Autodesk Inventor part; units mm, degrees
ref_plane "YZ Plane" through (0, 0, 0) normal (1, 0, 0) x (0, 1, 0)
ref_plane "XZ Plane" through (0, 0, 0) normal (0, 1, 0) x (-1, 0, 0)
ref_plane "XY Plane" through (0, 0, 0) normal (0, 0, 1) x (1, 0, 0)
sketch "Sketch1" plane through (0, 0, 0) normal (0, 0, 1) x (1, 0, 0)
  circle A0 centre (0, 0) radius 31
  circle A1 centre (0, 0) radius 34.175
  dimension "d0" = 62
  dimension "d1" = 68.35
extrude "Extrusion1" add sketch "Sketch1" along normal blind 6.35
ref_plane "Work Plane1" through (0, 0, -83.5) normal (0, 0, -1) x (-1, 0, 0)
sketch "Sketch2" plane through (0, 0, -83.5) normal (0, 0, -1) x (-1, 0, 0)
  circle A0 centre (0, 0) radius 30
  circle A1 centre (0, 0) radius 33.175
  circle A2 centre (0, 0) radius 23
  circle A3 centre (0, 0) radius 26.175
  dimension "d5" = 60
  dimension "d6" = 66.35
  dimension "d28" = 46
  dimension "d29" = 52.35
ref_plane "Work Plane2" through (0, 0, -57.65) normal (0, 0, -1) x (-1, 0, 0)
sketch "Sketch3" plane through (0, 0, -57.65) normal (0, 0, -1) x (-1, 0, 0)
  circle A0 centre (0, 0) radius 34.175
  circle A1 centre (0, 0) radius 31
  circle A2 centre (0, 0) radius 24
  circle A3 centre (0, 0) radius 27.175
  line L0 (0, 0) -> (34.175, 0)
  line L1 (0, 0) -> (34.175, 0) construction
  line L2 (0, 0) -> (33.8826, 4.4607)
  line L3 (0, 0) -> (33.8826, -4.4607)
  line L4 (33.8826, 4.4607) -> (33.8826, -4.4607)
  line L5 (33.8826, -4.4607) -> (0, -4.4607)
  line L6 (0, -4.4607) -> (0, 4.4607)
  line L7 (0, 4.4607) -> (33.8826, 4.4607)
  line L8 (33.8826, 4.4607) -> (33.8826, -4.4607)
  line L9 (33.8826, -4.4607) -> (37.0576, -4.4607)
  line L10 (37.0576, -4.4607) -> (37.0576, 4.4607)
  line L11 (37.0576, 4.4607) -> (33.8826, 4.4607)
  line L12 (-3.8631, 2.2304) -> (13.0782, 31.5736)
  line L13 (20.8044, 27.1129) -> (3.8631, -2.2304)
  line L14 (20.8044, 27.1129) -> (22.3919, 29.8625)
  line L15 (14.6657, 34.3232) -> (13.0782, 31.5736)
  line L16 (-3.8631, -2.2304) -> (-20.8044, 27.1129)
  line L17 (-13.0782, 31.5736) -> (3.8631, 2.2304)
  line L18 (-13.0782, 31.5736) -> (-14.6657, 34.3232)
  line L19 (-22.3919, 29.8625) -> (-20.8044, 27.1129)
  line L20 (0, -4.4607) -> (-33.8826, -4.4607)
  line L21 (-33.8826, 4.4607) -> (0, 4.4607)
  line L22 (-33.8826, 4.4607) -> (-37.0576, 4.4607)
  line L23 (-37.0576, -4.4607) -> (-33.8826, -4.4607)
  line L24 (3.8631, -2.2304) -> (-13.0782, -31.5736)
  line L25 (-20.8044, -27.1129) -> (-3.8631, 2.2304)
  line L26 (-20.8044, -27.1129) -> (-22.3919, -29.8625)
  line L27 (-14.6657, -34.3232) -> (-13.0782, -31.5736)
  line L28 (3.8631, 2.2304) -> (20.8044, -27.1129)
  line L29 (13.0782, -31.5736) -> (-3.8631, -2.2304)
  line L30 (13.0782, -31.5736) -> (14.6657, -34.3232)
  line L31 (22.3919, -29.8625) -> (20.8044, -27.1129)
  line L32 (-34.175, 6.35) -> (0, 6.35)
  line L33 (0, 6.35) -> (0, -6.35)
  line L34 (0, -6.35) -> (-34.175, -6.35)
  line L35 (-34.175, -6.35) -> (-34.175, 6.35)
  line L36 (-9.525, 34.175) -> (9.525, 34.175)
  line L37 (9.525, 34.175) -> (9.525, 0)
  line L38 (9.525, 0) -> (-9.525, 0)
  line L39 (-9.525, 0) -> (-9.525, 34.175)
  point P0 (-26.8064, 4.4607)
  point P1 (-33.8826, 4.4607)
  point P2 (-33.8826, -4.4607)
  point P3 (-26.8064, -4.4607)
  point P4 (-17.2663, -20.9846)
  point P5 (-20.8044, -27.1129)
  point P6 (-13.0782, -31.5736)
  point P7 (-9.5401, -25.4454)
  point P8 (9.5401, -25.4454)
  point P9 (20.8044, -27.1129)
  point P10 (17.2663, -20.9846)
  point P11 (26.8064, -4.4607)
  point P12 (26.8064, 4.4607)
  point P13 (17.2663, 20.9846)
  point P14 (20.8044, 27.1129)
  point P15 (13.0782, 31.5736)
  point P16 (9.5401, 25.4454)
  point P17 (-13.0782, 31.5736)
  point P18 (-20.8044, 27.1129)
  point P19 (-17.2663, 20.9846)
  point P20 (-9.5401, 25.4454)
  point P21 (-34.175, 0)
  point P22 (0, 0)
  point P23 (0, 0)
  point P24 (-7.9278, 22.6528)
  point P25 (-9.525, 25.4192)
  point P26 (-9.525, 29.5004)
  point P27 (9.525, 29.5004)
  point P28 (9.525, 25.4192)
  point P29 (7.9278, 22.6528)
  point P30 (-9.525, 22.0289)
  point P31 (9.525, 22.0289)
  dimension "d8" = 68.35
  dimension "d9" = 62
  dimension "d10" = 48
  dimension "d11" = 54.35
  dimension "d12" = 0
  dimension "d13" = 7.5
  dimension "d14" = 7.5
  dimension "d15" = 3.175
  dimension "d18" = 360
  dimension "d70" = 12.7
  dimension "d71" = 19.05
  dimension "d72" = 9.525
extrude "Extrusion2" add sketch "Sketch3" against normal up to surface (57.65 mm away) contours L0 L4 A0 | A0 L4 L0 | L7 A1 L13 A0 | L4 L0 A1 L2 | L2 A1 L7 | L5 A1 L3 | L3 A1 L0 L4 | A0 L28 A1 L5 | L13 A1 L12 A0 | A0 L29 A1 L28 | L12 A1 L37 A0 | A0 L24 A1 L29 | L37 A1 L39 A0 | A0 L25 A1 L24 | A0 L34 A1 L25 | L39 A1 L17 A0 | A0 L20 A1 L34 | L17 A1 L16 A0 | A0 L21 A1 L20 | L16 A1 L32 A0 | L32 A1 L21 A0
extrude "Extrusion3" add sketch "Sketch3" along normal blind 17 contours L2 A3 L7 A1 | A1 L0 A3 L2 | L7 A3 L13 A1 | L3 A3 L0 A1 | A1 L5 A3 L3 | A1 L28 A3 L5 | L13 A3 L12 A1 | L2 A2 L7 A3 | A3 L0 A2 L2 | L7 A2 L13 A3 | A1 L29 A3 L28 | L3 A2 L0 A3 | A3 L5 A2 L3 | A3 L28 A2 L5 | L12 A3 L37 A1 | L13 A2 L37 L12 A3 | A1 L24 A3 L29 | A3 L29 A2 L28 | L12 L37 A3 | A1 L25 A3 L24 | A3 L24 A2 L29 | L39 A3 L17 A1 | A1 L34 A3 L25 | A3 L25 A2 L24 | L17 A3 L16 A1 | L39 L17 A3 | A1 L20 A3 L34 | A3 L34 A2 L25 | L16 A3 L32 A1 | L17 L39 A2 L16 A3 | A1 L21 A3 L20 | A3 L20 A2 L34 | L32 A3 L21 A1 | L16 A2 L32 A3 | A3 L21 A2 L20 | L32 A2 L21 A3
extrude "Extrusion5" add sketch "Sketch3" along normal blind 6.35 contours L0 L4 A0 | A0 L4 L0 | L7 A1 L13 A0 | L4 L0 A1 L2 | L2 A1 L7 | L5 A1 L3 | L3 A1 L0 L4 | A0 L28 A1 L5 | L13 A1 L12 A0 | A0 L29 A1 L28 | L12 A1 L37 A0 | A0 L24 A1 L29 | L37 A1 L39 A0 | A0 L25 A1 L24 | A0 L34 A1 L25 | L39 A1 L17 A0 | A0 L20 A1 L34 | L17 A1 L16 A0 | A0 L21 A1 L20 | L16 A1 L32 A0 | L32 A1 L21 A0
sketch "Sketch4" plane through (0, 0, 6.35) normal (0, 0, 1) x (1, 0, 0)
  circle A0 centre (0, 0) radius 32
  line L0 (32, 25.4) -> (32, -25.4)
  line L1 (32, -25.4) -> (-69.6, -25.4)
  line L2 (-69.6, -25.4) -> (-69.6, 25.4)
  line L3 (-69.6, 25.4) -> (32, 25.4)
  circle A1 centre (0, 0) radius 31
  circle A2 centre (0, 0) radius 31
  circle A3 centre (0, 0) radius 34.175
  circle A4 centre (0, 0) radius 34.175
  point P0 (22.8642, 25.4)
  point P1 (-22.8642, 25.4)
  point P2 (-22.8642, -25.4)
  point P3 (22.8642, -25.4)
  point P4 (32, 11.9971)
  point P5 (32, -11.9971)
  dimension "d41" = 64
  dimension "d42" = 25.4
  dimension "d43" = 50.8
  dimension "d44" = 101.6
extrude "Extrusion7" add sketch "Sketch4" against normal up to surface (70.35 mm away) contours A0 L1 A1 L3 | L0 A3 L1 A0 | A0 L3 A3 L0 | L3 A1 A0 | A0 L3 A3 | L1 A3 A0 | A0 L1 A1 | A3 L3 L0 | L0 L1 A3 | L3 A1 L1 A0 | A0 L1 A3 L3 | A3 L1 L2 L3
extrude "Extrusion8" cut sketch "Sketch4" against normal through all contours L0 A3
sketch "Sketch8" plane through (-69.6, 25.4, 6.35) normal (0, 1, 0) x (1, 0, 0)
  circle A0 centre (12.7, 12.7) radius 2.5797
  line L0 (0, 0) -> (0, 70.35)
  line L1 (0, 0) -> (12.7, 0)
  line L2 (0, 0) -> (12.7, 0) construction
  line L3 (0, 0) -> (0, 12.7)
  line L4 (0, 0) -> (12.7, 0) construction
  circle A1 centre (25.4, 12.7) radius 2.5797
  circle A2 centre (12.7, 57.65) radius 2.5797
  circle A3 centre (25.4, 57.65) radius 2.5797
  line L5 (46.7358, 0) -> (0, 0)
  line L6 (46.7358, 70.35) -> (0, 70.35)
  point P0 (69.6, 6.35)
  dimension "d73" = 12.7
  dimension "d74" = 0
  dimension "d75" = 12.7
  dimension "d76" = 90
  dimension "d79" = 12.7
  dimension "d82" = 44.95
  dimension "d85" = 5.1594
  dimension "d86" = 12.7
  dimension "d87" = 12.7
  dimension "d88" = 12.7
extrude "Extrusion11" cut sketch "Sketch8" against normal through all
equation "\"d14\" = d13"
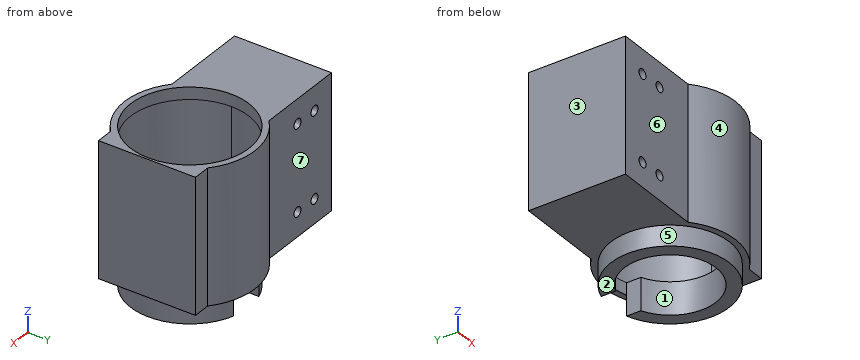
Could you check a few things on this model? Use its own coordinates, in mm. Face numbers are marked on the shaded views. A direction names the side the tool comes from. Round coordinates to 2 decimals unless told otherwise and drop trailing zeros. Write each loop counter-clockwise with the first axis right and the second up, starting at its lowest first coordinate (ties: lowest second). Pieces come first, ordered by that corner, then holes. Notation, with made-up numbers: (-34.75, 37) -> (17.25, 37) arc R23 cw to (17.25, 65) -> close; hole circle Ø2 at (-24, 41.25). An arc over 180 degrees is marked (long way). Use a Markdown table: item, result.
1. If we section it at D-D (x = 0): List the corners of the cut face in (y, z) for me (3 decimals).
Answer key:
| item | result |
|---|---|
| outline | (-34.175, -64) -> (-31, -64) -> (-31, -74.65) -> (-24, -74.65) -> (-24, -57.65) -> (-31, -57.65) -> (-31, 6.35) -> (-34.175, 6.35) -> close; (31, -64) -> (34.175, -64) -> (34.175, 6.35) -> (31, 6.35) -> close |
2. For pin 1 Ø3.5 at (y, z) = (27.5, -68) entering from -X; pin 2 Ø4.5 at (x, z) = (25.5, -24.5) entering from +Y; pin 3 Ø2 at (y, z) = (24.5, -66) entering from +X, each with a flat end and sliding along its axis, tell me the tip position at first contact or that it passes through.
Answer key:
| item | result |
|---|---|
| pin 1 | stops at x = -17.26 |
| pin 2 | stops at y = 25.4 |
| pin 3 | stops at x = 20.22 |
3. Which directions (+Z, -Z, +X, -X, +Y, -Y) give clear straight access to the entire face, cutting with the end or side of a thin tool? Please do the marked faces 4, 5, 6 and 7.
Answer key:
| item | result |
|---|---|
| face 4 | +Z, -Z, -Y |
| face 5 | -Z |
| face 6 | +Z, -Z, -X, -Y |
| face 7 | +Z, -Z, -X, +Y |
4. If we section it at C-C (y = -18): List the corners of the cut face in (x, z) for me, then the cut area to 3 significant figures.
Answer key:
| item | result |
|---|---|
| outline | (-69.6, -64) -> (-25.24, -64) -> (-25.24, -74.65) -> (-15.87, -74.65) -> (-15.87, -57.65) -> (-25.24, -57.65) -> (-25.24, 6.35) -> (-69.6, 6.35) -> close; (15.87, -74.65) -> (25.24, -74.65) -> (25.24, -64) -> (32, -64) -> (32, 6.35) -> (25.24, 6.35) -> (25.24, -57.65) -> (15.87, -57.65) -> close; hole circle Ø5.16 at (-56.9, -51.3); hole circle Ø5.16 at (-56.9, -6.35); hole circle Ø5.16 at (-44.2, -51.3); hole circle Ø5.16 at (-44.2, -6.35) |
| area | 3,830 mm^2 |
5. We'd pull the mould along X, two halves only. Please class the marked faces 1, 2 and 3: +X half, -X half, draft (parallel to the pull), parting line (faces both ways), or undercut.
Answer key:
| item | result |
|---|---|
| face 1 | undercut |
| face 2 | draft |
| face 3 | -X half |
6. Please list where these lines run through material, in increasing order: probe 1 along Z at (x, y) = (-56.9, 2); probe 2 along X at (y, z) = (0, -61); probe 3 along X at (y, z) = (0, -68.5).
Answer key:
| item | result |
|---|---|
| probe 1 | z = -64 to -53.88, -48.72 to -8.93, -3.77 to 6.35 |
| probe 2 | x = -69.6 to -24, 24 to 32 |
| probe 3 | x = -31 to -24, 24 to 31 |
7. If we section it at B-B (x = -56.9): List the corners of the cut face in (y, z) for me, then the cut area to 3 significant figures.
Answer key:
| item | result |
|---|---|
| outline | (-25.4, -64) -> (25.4, -64) -> (25.4, -53.88) -> (-25.4, -53.88) -> close; (-25.4, -48.72) -> (25.4, -48.72) -> (25.4, -8.93) -> (-25.4, -8.93) -> close; (-25.4, -3.77) -> (25.4, -3.77) -> (25.4, 6.35) -> (-25.4, 6.35) -> close |
| area | 3,050 mm^2 |
8. If we section it at A-A (z = -51.3): List the corners of the cut face in (x, y) for me (3 decimals).
Answer key:
| item | result |
|---|---|
| outline | (-69.6, -25.4) -> (-59.48, -25.4) -> (-59.48, 25.4) -> (-69.6, 25.4) -> close; (-54.32, -25.4) -> (-46.78, -25.4) -> (-46.78, 25.4) -> (-54.32, 25.4) -> close; (-41.62, -25.4) -> (-22.864, -25.4) arc R34.175 ccw to (22.864, -25.4) -> (32, -25.4) -> (32, 25.4) -> (22.864, 25.4) arc R34.175 ccw to (-22.864, 25.4) -> (-41.62, 25.4) -> close; hole circle Ø62 at (0, 0) |
